Read the model definition and answer for the solid it produces. Units are mm, in the model's axes. Face numbers are marked on the shaded views. Coordinates: 2 decimals unless noted, no trailing zeros. Write each loop counter-clockwise with the first axis right and the second up, starting at its lowest first coordinate (ties: lowest second). Pieces come first, ordered by that corner, then holes. Notation, with made-up numbers: (14, 59) -> (59, 59) arc R18 ccw to (59, 78) -> close; hole circle Ø1 at (-31, 38.25). An arc over 180 degrees is marked (long way). One line per item, written item: value. Start each with the question number.
1. Find section C-C, the plane z = 55. Write down the section's boundary in (x, y).
2. Find section B-B, the plane z = 83.5. Write down the section's boundary in (x, y).
3. Given P1, Ø10, axis at y = 68, z = 83, coming from the +X side; P2, Ø4, axis at x = 0, z = 114.3, coming from the -Y side; P3, Ø2, axis at y = 96.5, z = 106, coming from the +X side; P4, Ø3, axis at x = 44.5, y = 265, coming from the -Z side, each flat-ended and moving along its own axis, determine where each tip first touches the part or whether it passes through.
4. For a pull along Z with two mould halves and no side action, classify the marked faces 1, 2, 3 and 4 as pulls with the +Z half, pulls with the -Z half, needs draft (parallel to the pull), parting line crosses it, or undercut.
5. Find section A-A, the plane y = 50. State how many separate pieces and enclosed holes the cut face has, and give its area (3 significant figures).
6. Consider line 1 along X through (y, z) = (260, 100.5); line 2 along X through (y, z) = (147, 114); line 3 along Z through (x, y) = (-1, 57). Determine where each line is inside the solid, lowest interval first.
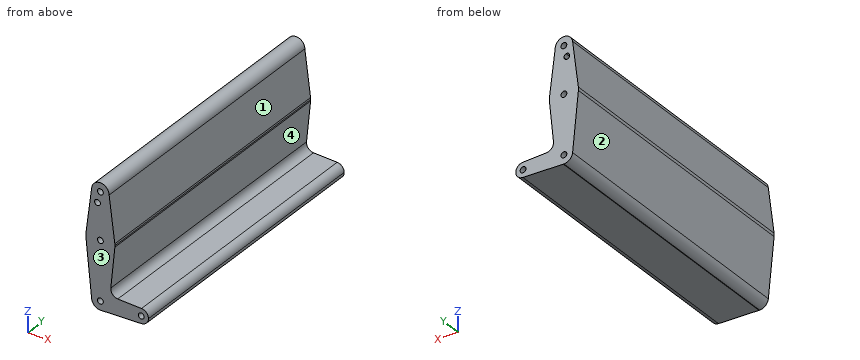
```python
from build123d import *

# Parameters (mm, degrees)
F0_R     = 3.175
F1_DEPTH = 304.8


with BuildPart() as f1:
    # F0 (on Front) → F1 (new body)
    with BuildSketch(Plane.XZ):
        with BuildLine():
            ThreePointArc((-2.3812504012, 105.0774585104), (5.8328472862, 106.7698261948), (9.525, 114.3))
            ThreePointArc((9.525, 114.3), (0.596483242, 123.8063048942), (-9.4502929642, 115.490625))
            ThreePointArc((-9.4502929642, 115.490625), (-7.8806639116, 108.9501624966), (-2.3812504012, 105.0774585104))
        make_face()
        with Locations((0, 114.3)):
            Circle(F0_R, mode=Mode.SUBTRACT)
        with BuildLine():
            Line((15.7474569047, 65.5082893304), (9.525, 114.3))
            ThreePointArc((9.525, 114.3), (5.8328472862, 106.7698261948), (-2.3812504012, 105.0774585104))
            ThreePointArc((-2.3812504012, 105.0774585104), (-7.8806639116, 108.9501624966), (-9.4502929642, 115.490625))
            Line((-9.4502929642, 115.490625), (-15.7504882737, 65.484375))
            ThreePointArc((-15.7504882737, 65.484375), (-0.0120528461, 79.3749954245), (15.7474569047, 65.5082893304))
        make_face()
        with BuildLine():
            ThreePointArc((0, 102.0032778758), (-5.6850577659, 100.0589952287), (-2.3812504012, 105.0774585104))
            ThreePointArc((-2.3812504012, 105.0774585104), (-0.6649422341, 103.9475605229), (0, 102.0032778758))
        make_face(mode=Mode.SUBTRACT)
        with BuildLine():
            ThreePointArc((15.875, 63.5), (15.8430821396, 64.5061676396), (15.7474569047, 65.5082893304))
            ThreePointArc((15.7474569047, 65.5082893304), (-0.0120528461, 79.3749954245), (-15.7504882737, 65.484375))
            ThreePointArc((-15.7504882737, 65.484375), (-15.8737438155, 63.6997054867), (-15.7954255641, 61.9125))
            ThreePointArc((-15.7954255641, 61.9125), (0, 47.625), (15.7954255641, 61.9125))
            ThreePointArc((15.7954255641, 61.9125), (15.8550939106, 62.7052534459), (15.875, 63.5))
        make_face()
        with Locations((0, 63.5)):
            Circle(F0_R, mode=Mode.SUBTRACT)
        with BuildLine():
            ThreePointArc((15.7954255641, 61.9125), (0, 47.625), (-15.7954255641, 61.9125))
            Line((-15.7954255641, 61.9125), (-9.4772553384, -0.9525))
            ThreePointArc((-9.4772553384, -0.9525), (-0.4768479324, 9.5130563464), (9.525, 0))
            ThreePointArc((9.525, 0), (6.9705567315, -6.4912990883), (0.6773435479, -9.500885786))
            Line((0.6773435479, -9.500885786), (44.7324052746, -7.9324746146))
            ThreePointArc((44.7324052746, -7.9324746146), (36.5125, 0), (44.7324052746, 7.9324746146))
            Line((44.7324052746, 7.9324746146), (18.968327868, 8.8497055806))
            ThreePointArc((18.968327868, 8.8497055806), (13.2612039825, 11.5674628959), (11.3408358685, 17.5898921545))
            Line((11.3408358685, 17.5898921545), (15.7954255641, 61.9125))
        make_face()
        with BuildLine():
            ThreePointArc((9.525, 0), (-0.4768479324, 9.5130563464), (-9.4772553384, -0.9525))
            ThreePointArc((-9.4772553384, -0.9525), (-6.3895642457, -7.063929059), (0, -9.525))
            Line((0, -9.525), (0.6773435479, -9.500885786))
            ThreePointArc((0.6773435479, -9.500885786), (6.9705567315, -6.4912990883), (9.525, 0))
        make_face()
        Circle(F0_R, mode=Mode.SUBTRACT)
        with BuildLine():
            Line((0.6773435479, -9.500885786), (0, -9.525))
            ThreePointArc((0, -9.525), (0.3388863295, -9.5189695375), (0.6773435479, -9.500885786))
        make_face()
        with BuildLine():
            ThreePointArc((52.3875, 0), (50.1616327839, 5.5119104847), (44.7324052746, 7.9324746146))
            ThreePointArc((44.7324052746, 7.9324746146), (36.5125, 0), (44.7324052746, -7.9324746146))
            ThreePointArc((44.7324052746, -7.9324746146), (50.1616327839, -5.5119104847), (52.3875, 0))
        make_face()
        with Locations((44.45, 0)):
            Circle(F0_R, mode=Mode.SUBTRACT)
    extrude(amount=-F1_DEPTH)


solid = f1.part
```
Answer block:
1. outline: (-15.1, 0) -> (15.1, 0) -> (15.1, 304.8) -> (-15.1, 304.8) -> close
2. outline: (-13.48, 0) -> (13.45, 0) -> (13.45, 304.8) -> (-13.48, 304.8) -> close
3. P1: stops at x = 14.15
3. P2: passes through
3. P3: stops at x = 10.71
3. P4: stops at z = -7.99
4. face 1: pulls with the +Z half
4. face 2: pulls with the -Z half
4. face 3: needs draft
4. face 4: undercut
5. separate pieces: 1
5. enclosed holes: 5
5. area: 3,770 mm2
6. line 1: x = -11.34 to -5.97, -0.38 to 11.28
6. line 2: x = -9.64 to -3.16, 3.16 to 9.56
6. line 3: z = -9.47 to -3.01, 3.01 to 60.49, 66.51 to 99.69, 104.32 to 111.29, 117.31 to 123.77
